Read the model definition and answer for the solid it produces. Units are mm, in the model's axes. Face numbers are marked on the shaded views. A direction names the side the tool comes from. Give positions to 0.01 mm unless a question says otherwise; leave off trailing zeros. Loops run counter-clockwise (first coordinate to the right, second up) from the corner with the lowest first, then second, coordinate; pieces in that order, holes last. Notation, with made-up numbers: M 56.25,-2.5 L 67.25,-2.5 A30 cw 67.25,30.5 Z; hole C 73,18.5 d4. An arc over 180 degrees is marked long. Return JSON: item names as keys, results as strings. Group by question number.
Autodesk Inventor part; units mm, degrees
ref_plane "YZ Plane" through (0, 0, 0) normal (1, 0, 0) x (0, 1, 0)
ref_plane "XZ Plane" through (0, 0, 0) normal (0, 1, 0) x (-1, 0, 0)
ref_plane "XY Plane" through (0, 0, 0) normal (0, 0, 1) x (1, 0, 0)
sketch "Sketch1" plane through (0, 0, 0) normal (0, 1, 0) x (-1, 0, 0)
  line L0 (58.8, 0) -> (0, 0)
  line L1 (0, 0) -> (0, -32)
  line L2 (0, -32) -> (58.8, -32)
  line L3 (58.8, -32) -> (58.8, 0)
  line L4 (41.9, -3.5) -> (16.9, -3.5) construction
  line L5 (16.9, -3.5) -> (16.9, -28.5) construction
  line L6 (16.9, -28.5) -> (41.9, -28.5) construction
  line L7 (41.9, -28.5) -> (41.9, -3.5) construction
  circle A0 centre (41.9, -3.5) radius 1.5
  circle A1 centre (16.9, -3.5) radius 1.5
  circle A2 centre (41.9, -28.5) radius 1.5
  circle A3 centre (16.9, -28.5) radius 1.5
  point P0 (41.9, -16)
  point P1 (58.8, -16)
  point P2 (29.4, -28.5)
  point P3 (29.4, -32)
  dimension "d0" = 3
  dimension "d1" = 25
  dimension "d2" = 32
  dimension "d3" = 58.8
extrude "Extrusion1" add sketch "Sketch1" along normal blind 2
sketch "Sketch2" plane through (-58.8, 0, -32) normal (-1, 0, 0) x (0, 0, 1)
  circle A0 centre (31, 17.2) radius 16 construction
  circle A1 centre (42.3137, 28.5137) radius 2.4
  circle A2 centre (15, 17.2) radius 2.4
  circle A3 centre (19.6863, 5.8863) radius 2.4
  circle A4 centre (19.6863, 28.5137) radius 2.4
  circle A5 centre (47, 17.2) radius 2.4
  circle A6 centre (42.3137, 5.8863) radius 2.4
  line L0 (19.6863, 28.5137) -> (42.3137, 5.8863) construction
  line L1 (15, 17.2) -> (31, 17.2) construction
  line L2 (0, 2) -> (32, 2)
  arc A7 (43.0482, 0) -> (16.51, 2) centre (31, 17.2) ccw
  line L3 (0, 0) -> (32, 0)
  line L4 (32, 0) -> (43.0482, 0)
  line L5 (32, 0) -> (32, 2)
  line L6 (0, 2) -> (0, 38.2)
  line L7 (0, 38.2) -> (31, 38.2)
  circle A8 centre (31, 17.2) radius 6.25
  point P0 (31, 17.2)
  dimension "d6" = 4.8
  dimension "d7" = 32
  dimension "d9" = 15.2
  dimension "d11" = 45
  dimension "d12" = 31
  dimension "d14" = 21
  dimension "d17" = 12.5
extrude "Extrusion2" add sketch "Sketch2" against normal up to surface (58.8 mm away)
sketch "Sketch3" plane through (-58.8, 0, -32) normal (-1, 0, 0) x (0, 0, 1)
  circle A0 centre (31, 17.2) radius 10.025
  circle A1 centre (31, 17.2) radius 6.25 construction
  point P0 (32, 0)
  dimension "d18" = 20.05
extrude "Extrusion3" cut sketch "Sketch3" against normal blind 27.05
sketch "Sketch4" plane through (-58.8, 38.2, -1) normal (0, 1, 0) x (1, 0, 0)
  circle A0 centre (41.9, 2.5) radius 1.5
  circle A1 centre (41.9, 27.5) radius 1.5
  circle A2 centre (16.9, 2.5) radius 1.5
  circle A3 centre (16.9, 27.5) radius 1.5
  circle A4 centre (16.9, 2.5) radius 3
  circle A5 centre (16.9, 27.5) radius 3
  circle A6 centre (41.9, 27.5) radius 3
  circle A7 centre (41.9, 2.5) radius 3
  point P0 (58.8, -1)
  dimension "d21" = 6
extrude "Extrusion4" cut sketch "Sketch4" against normal up to surface (36.2 mm away) contours A0 | A1 | A2 | A3 | A4 | A5 | A6 | A7
properties part number "X_Axis_Connector"
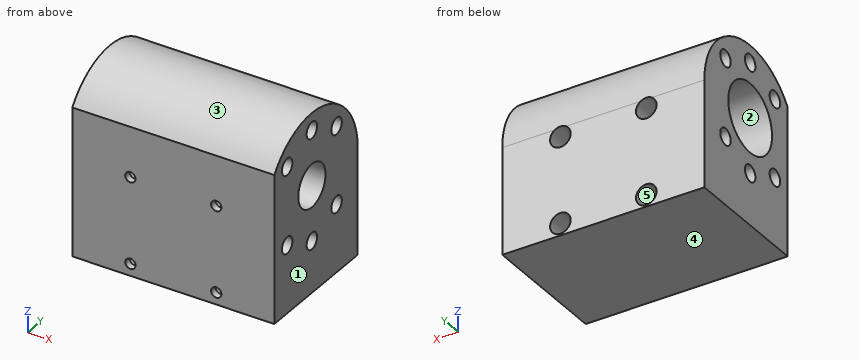
1. Straight lines are drawn through the part: line 1 along Y through (x, z) = (-18, -17); line 2 along Y through (x, z) = (-10.5, 11); line 3 along Y through (x, z) = (-49, 12). For each, find the intervals that lie inside material, in ascending order.
2. The mould has two halves that part along Z. Classify the marked faces 1, 2 and 3: +Z half, -Z half, draft (parallel to the pull), parting line (faces both ways), or undercut.
3. For the marked faces 4 and 5, determine the directions among +Z, -Z, +X, -X, +Y, -Y from which every point of the face is accessible in a straight line to the end or side of a thin tool.
4. Flat-ended cylindrical pins translate along their axes: P1, Ø5.5, axis at x = -41.9, z = -3.5, coming from the +Y side; P2, Ø8, axis at x = -45, z = 12, coming from the +Y side; P3, Ø4, axis at y = 17.2, z = 15, coming from the -X side; P4, Ø5, axis at x = -12, y = 11.5, coming from the +Z side. Find the tip coordinate at first contact, or state that the pin passes through.
5. Find section D-D (z = -28.5). Write down the section's boundary in (x, y).
6. Find section C-C (x = -16.9). State how many separate pieces and enclosed holes the cut face has, and give its area (3 significant figures).
7. Find section B-B (z = -17). Write down the section's boundary in (x, y), and give its area (3 significant figures).
8. Find section A-A (y = 17.2). Write down the section's boundary in (x, z) (3 decimals).
Result:
{
 "1": {"line 1": "y = 0 to 14.8, 19.6 to 38.2", "line 2": "y = 0 to 3.59, 8.19 to 26.21, 30.81 to 34.43", "line 3": "y = 0.71 to 4.18, 7.59 to 26.81, 30.22 to 33.69"},
 "2": {"face 1": "draft", "face 2": "undercut", "face 3": "+Z half"},
 "3": {"face 4": "-Z, +X, -X, +Y, -Y", "face 5": "+Y"},
 "4": {"P1": "stops at y = 2", "P2": "stops at y = 36.17", "P3": "passes through", "P4": "stops at z = 19.75"},
 "5": {"outline": "M -58.8,0 L -43.4,0 L -43.4,2 L -44.9,2 L -44.9,38.2 L -58.8,38.2 Z; M -40.4,0 L -18.4,0 L -18.4,2 L -19.9,2 L -19.9,38.2 L -38.9,38.2 L -38.9,2 L -40.4,2 Z; M -15.4,0 L 0,0 L 0,38.2 L -13.9,38.2 L -13.9,2 L -15.4,2 Z"},
 "6": {"separate pieces": "3", "enclosed holes": "6", "area": "1,230 mm2"},
 "7": {"outline": "M -58.8,0 L 0,0 L 0,14.8 L -58.8,14.8 Z; M -58.8,19.6 L 0,19.6 L 0,38.2 L -58.8,38.2 Z", "area": "1,960 mm2"},
 "8": {"outline": "M -58.8,-32 L 0,-32 L 0,-19.4 L -58.8,-19.4 Z; M -58.8,-14.6 L 0,-14.6 L 0,-7.25 L -31.75,-7.25 L -31.75,-11.025 L -58.8,-11.025 Z; M -58.8,9.025 L -31.75,9.025 L -31.75,5.25 L 0,5.25 L 0,12.6 L -58.8,12.6 Z; M -58.8,17.4 L 0,17.4 L 0,20 L -58.8,20 Z; hole C -41.9,-28.5 d6; hole C -16.9,-28.5 d6"}
}
